Could you check a few things on this model? Use its own coordinates, in mm. Face numbers are marked on the shaded views. Round coordinates to 2 decimals unless told otherwise and drop trailing zeros. Loops run counter-clockwise (first coordinate to the right, second up) from the corner with the lowest first, then second, coordinate; pieces in that order, holes last.
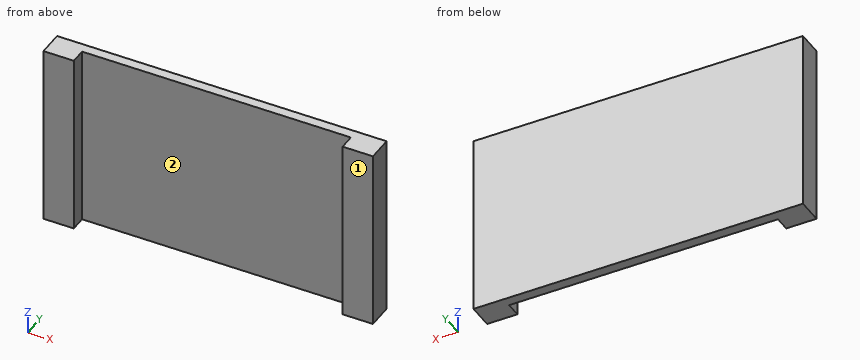
from build123d import *

# Parameters (mm, degrees)
SKETCH1_W           = 33.15
SKETCH1_H           = 18.5
BOSS_EXTRUDE1_DEPTH = 2.55
SKETCH2_W           = 27.05
SKETCH2_H           = 18.5
CUT_EXTRUDE1_DEPTH  = 1.55


with BuildPart() as part:
    # Sketch1 → Boss-Extrude1 (new body)
    with BuildSketch(Plane(origin=(0, 0, 0), x_dir=(1, 0, 0), z_dir=(0, 1, 0))):
        Rectangle(SKETCH1_W, SKETCH1_H)
    extrude(amount=BOSS_EXTRUDE1_DEPTH)

    # Sketch2 → Cut-Extrude1 (cut)
    with BuildSketch(Plane.XZ):
        Rectangle(SKETCH2_W, SKETCH2_H)
    extrude(amount=-CUT_EXTRUDE1_DEPTH, mode=Mode.SUBTRACT)


solid = part.part
Item 1: If we section it at C-C, the plane x = 8: Please give me the cut outline in (y, z).
Results list:
outline: (1.55, -9.25) - (2.55, -9.25) - (2.55, 9.25) - (1.55, 9.25) - close
Item 2: If we section it at B-B, the plane z = 1: Please give me the cut outline in (x, y) (3 decimals), then the cut area to 3 significant figures.
Results list:
outline: (-16.575, 0) - (-13.525, 0) - (-13.525, 1.55) - (13.525, 1.55) - (13.525, 0) - (16.575, 0) - (16.575, 2.55) - (-16.575, 2.55) - close
area: 42.6 mm2
Item 3: If we section it at A-A, the plane y = 0.45: Please give me the cut outline in (x, z) (3 decimals), then the cut area to 3 significant figures.
Results list:
outline: (-16.575, -9.25) - (-13.525, -9.25) - (-13.525, 9.25) - (-16.575, 9.25) - close; (13.525, -9.25) - (16.575, -9.25) - (16.575, 9.25) - (13.525, 9.25) - close
area: 113 mm2
Item 4: If I drill on line 1 along X through (y, z) = (0.4, 5) (3 decimals); line 2 along Y through (x, z) = (9, -4.5), over which ranges is the centre line in solid material (lowest first)?
Results list:
line 1: x = -16.575 to -13.525, 13.525 to 16.575
line 2: y = 1.55 to 2.55
Item 5: Will this pin go through, and if not, where does the flat tip stop? pin 1 (5.5 mm diameter, centred on x = -2, z = 3, fed in from -Y).
Results list:
pin 1: stops at y = 1.55
Item 6: We'd pull the mould along X, two halves only. Please class the marked faces 1 and 2: released by +X, released by -X, zero draft, split by the parting line, or undercut.
Results list:
face 1: zero draft
face 2: undercut
